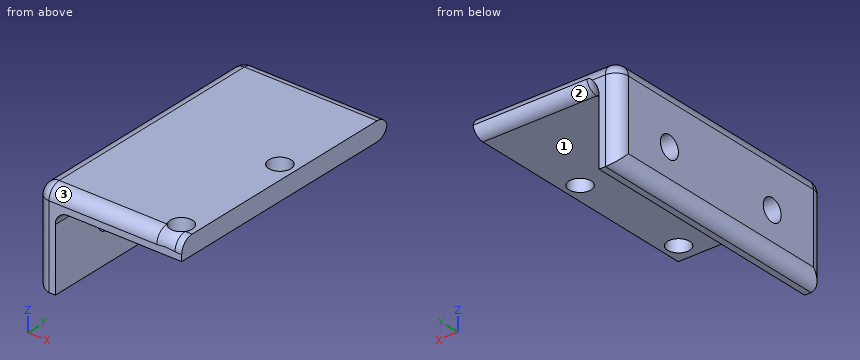
Autodesk Inventor part; units mm, degrees
ref_plane "YZ Plane" through (0, 0, 0) normal (1, 0, 0) x (0, 1, 0)
ref_plane "XZ Plane" through (0, 0, 0) normal (0, 1, 0) x (-1, 0, 0)
ref_plane "XY Plane" through (0, 0, 0) normal (0, 0, 1) x (1, 0, 0)
sketch "Sketch1" plane through (0, 0, 0) normal (0, 1, 0) x (-1, 0, 0)
  line L0 (-10, 1.5) -> (10, 1.5)
  line L1 (10, 1.5) -> (10, -1.5)
  line L2 (10, -1.5) -> (-10, -1.5)
  line L3 (-10, -1.5) -> (-10, 1.5)
  line L4 (-10, 1.5) -> (10, -1.5) construction
  line L5 (10, 1.5) -> (-10, -1.5) construction
  line L6 (10, 1.5) -> (10, -13.5)
  line L7 (10, -13.5) -> (13, -13.5)
  line L8 (13, -13.5) -> (13, 1.5)
  line L9 (13, 1.5) -> (10, 1.5)
  point P0 (0, 0)
  dimension "d0" = 20
  dimension "d1" = 3
  dimension "d2" = 15
  dimension "d3" = 3
extrude "Extrusion1" add sketch "Sketch1" along normal blind 40
sketch "Sketch2" plane through (10, 0, -1.5) normal (0, 0, -1) x (-1, 0, 0)
  line L0 (0, 0) -> (23, 0)
  line L1 (0, 0) -> (2.5, 0)
  line L2 (2.5, 0) -> (2.5, 3)
  line L3 (2.5, 0) -> (5.5, 0) construction
  circle A0 centre (2.5, 3) radius 1.75
  line L4 (2.5, 3) -> (2.5, 22.175)
  line L5 (2.5, 3) -> (21.675, 3) construction
  circle A1 centre (2.5, 22.175) radius 1.75
  point P0 (10, 0)
  dimension "d6" = 2.5
  dimension "d7" = 3
  dimension "d8" = 90
  dimension "d9" = 3.5
  dimension "d10" = 19.175
  dimension "d11" = 90
  dimension "d12" = 3.5
extrude "Extrusion2" cut sketch "Sketch2" against normal blind 3
fillet "Fillet1" radius 2 3 edges at (-13, 20, -13.5) (-13, 0, -6) (-13, 40, -6)
fillet "Fillet2" radius 2 4 edges at (0, 40, -1.5) (-13, 20, 1.5) (-0.5, 0, 1.5) (-0.5, 40, 1.5)
fillet "Fillet3" radius 2 2 edges at (-10, 39.2247, -1.0811) (-10, 19, -1.5)
sketch "Sketch3" plane through (-13, 2, -11.5) normal (-1, 0, 0) x (0, 0, 1)
  line L0 (-2, -2) -> (-2, 38)
  line L1 (-2, -2) -> (-2, 18)
  line L2 (-2, 18) -> (4.5, 18)
  line L3 (-2, -2) -> (11, -2)
  line L4 (4.5, 18) -> (4.5, 8)
  line L5 (4.5, 18) -> (14.5, 18) construction
  line L6 (4.5, 18) -> (4.5, 28)
  line L7 (4.5, 18) -> (14.5, 18) construction
  circle A0 centre (4.5, 8) radius 1.75
  circle A1 centre (4.5, 28) radius 1.75
  point P0 (11.5, -2)
  dimension "d18" = 10
  dimension "d19" = 90
  dimension "d20" = 6.5
  dimension "d21" = 10
  dimension "d22" = 90
  dimension "d23" = 3.5
  dimension "d24" = 3.5
extrude "Extrusion3" cut sketch "Sketch3" against normal blind 3
properties part number "Limit_Switch_Bracket"
Source: CAD feature listing. Evaluate the final solid. Frame: model axes, mm. Face numbers are marked on the shaded views. A direction names the side the tool comes from. Give positions to 0.01 mm unless a question says otherwise; leave off trailing zeros. Write each loop counter-clockwise with the first axis right and the second up, starting at its lowest first coordinate (ties: lowest second). Pieces come first, ordered by that corner, then holes.
1. Section query B-B (z = -7). Return the cut outline in (x, y).
2. Section query A-A (y = 10). Return the cut outline in (x, z), then the cut area to 3 significant figures.
3. Section query C-C (x = 5). Return the cut outline in (y, z).
4. Section query D-D (y = 34.5). Return the cut outline in (x, z).
5. Material intervals for line 1 along Z through (x, y) = (-10.85, 10); line 2 along Y through (x, z) = (7.5, 0.65) (3 decimals); line 3 along Y through (x, z) = (7.5, 0.25) (3 decimals), sorted ascending.
6. First-contact query: pin 1 (4 mm diameter, centred on x = 7.5, y = 22.175, fed in from -Z); pin 2 (2 mm diameter, centred on y = 10, z = -7, fed in from +X); pin 3 (5.5 mm diameter, centred on y = 25, z = -9, fed in from +X). Flat tips, straight axial feed; report the tip coordinate or a pass-through.
7. Access query for the marked faces 1, 2 and 3. Directions: +Z, -Z, +X, -X, +Y, -Y. A direction counts if a zero-diameter tool reaches every point of the face in a straight line with its end or side. Return the directions, or none.
Output values:
1. outline: (-13, 2) arc R2 ccw to (-11, 0) - (-10, 0) - (-10, 8.25) - (-13, 8.25) - close; (-13, 11.75) - (-10, 11.75) - (-10, 28.25) - (-13, 28.25) - close; (-13, 31.75) - (-10, 31.75) - (-10, 40) - (-11, 40) arc R2 ccw to (-13, 38) - close
2. outline: (-13, -11.5) arc R2 ccw to (-11, -13.5) - (-10, -13.5) - (-10, -8.75) - (-13, -8.75) - close; (-13, -5.25) - (-10, -5.25) - (-10, -3.5) arc R2 cw to (-8, -1.5) - (10, -1.5) - (10, 1.5) - (-11, 1.5) arc R2 ccw to (-13, -0.5) - close
2. area: 93.6 mm2
3. outline: (0, -1.5) - (38, -1.5) arc R2 ccw to (39.94, 0) arc R2 ccw to (38, 1.5) - (2, 1.5) arc R2 ccw to (0, -0.5) - close
4. outline: (-13, -11.5) arc R2 ccw to (-11, -13.5) - (-10, -13.5) - (-10, -3.5) arc R2 cw to (-8, -1.5) - (10, -1.5) - (10, 1.5) - (-11, 1.5) arc R2 ccw to (-13, -0.5) - close
5. line 1: z = -13.5 to -8.75, -5.25 to 1.5
5. line 2: y = 0.27 to 1.25, 4.75 to 20.425, 23.925 to 39.636
5. line 3: y = 0.093 to 1.25, 4.75 to 20.425, 23.925 to 39.854
6. pin 1: stops at z = -1.5
6. pin 2: passes through
6. pin 3: stops at x = -10
7. face 1: -Z, +X, +Y, -Y
7. face 2: -Z, +X, +Y
7. face 3: +Z, -X, -Y
